```python
from build123d import *

# Parameters (mm, degrees)
SKETCH1_R           = 3.5
BOSS_EXTRUDE1_DEPTH = 30
SKETCH2_R           = 1.2
CUT_EXTRUDE1_DEPTH  = 15
SKETCH3_R           = 1.1
CUT_EXTRUDE2_DEPTH  = 15
CUT_EXTRUDE3_START  = -30
CUT_EXTRUDE3_DEPTH  = 30


with BuildPart() as part:
    # Sketch1 → Boss-Extrude1 (new body)
    with BuildSketch(Plane(origin=(0, 0, 0), x_dir=(0, 0, -1), z_dir=(1, 0, 0))):
        Circle(SKETCH1_R)
    extrude(amount=BOSS_EXTRUDE1_DEPTH)

    # Sketch2 → Cut-Extrude1 (cut)
    with BuildSketch(Plane.ZY):
        Circle(SKETCH2_R)
    extrude(amount=-CUT_EXTRUDE1_DEPTH, mode=Mode.SUBTRACT)

    # Sketch3 → Cut-Extrude2 (cut)
    with BuildSketch(Plane(origin=(30, 0, 0), x_dir=(0, 0, -1), z_dir=(1, 0, 0))):
        Circle(SKETCH3_R)
    extrude(amount=-CUT_EXTRUDE2_DEPTH, mode=Mode.SUBTRACT)

    # Sketch4 → Cut-Extrude3 (cut)
    with BuildSketch(Plane(origin=(30, 0, 0), x_dir=(0, 0, -1), z_dir=(1, 0, 0)).offset(CUT_EXTRUDE3_START)):
        with BuildLine():
            Line((2.449489743, 2.5), (2.449489743, -2.5))
            ThreePointArc((2.449489743, -2.5), (3.5, 0), (2.449489743, 2.5))
        make_face()
    extrude(amount=CUT_EXTRUDE3_DEPTH, mode=Mode.SUBTRACT)


solid = part.part
```
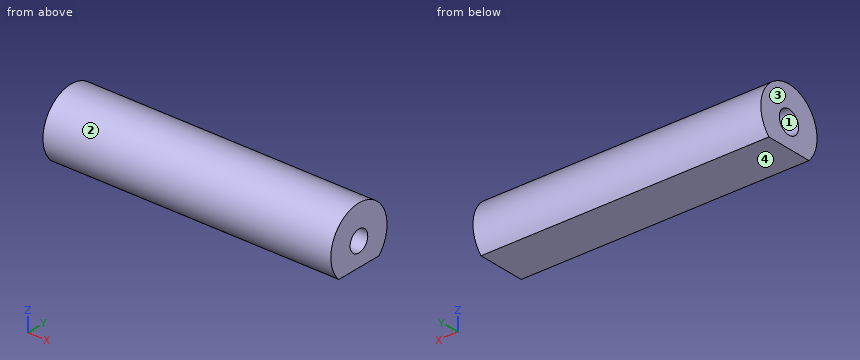
Input: part model. Units: mm. Frame: model coordinates. Face numbers are marked on the shaded views. Round coordinates to 2 decimals unless told otherwise and drop trailing zeros. Loops run counter-clockwise (first coordinate to the right, second up) from the corner with the lowest first, then second, coordinate; pieces in that order, holes last. Notation, with made-up numbers: (78.5, -37.75) -> (113.5, -37.75) arc R17 cw to (113.5, -16.75) -> close; hole circle Ø3 at (-25, 43). An arc over 180 degrees is marked (long way). Use one line per item in the form item = value. Start each with the question number.
Item 1: Section query A-A on z = 0. Return the cut outline in (x, y), then the cut area to 3 significant figures.
Item 2: Contact query for a flat-ended pin moving along its axis: pin 1 Ø2 at (x, z) = (9.5, 1.5) entering from -Y. Output: stop coordinate, or through.
Item 3: Section query C-C on x = 23.5. Return the cut outline in (y, z), then the cut area to 3 significant figures.
Item 4: Material intervals for L1, parallel to Y at x = 25.5, z = 0; L2, parallel to Y at x = 6.25, z = 0; L3, parallel to Z at x = 18, y = -0.25, sorted ascending. Write a range as from..to.
Item 5: Mould query, pull axis Z, two halves, no side actions, for the marked faces 1, 2, 3 and 4. Classes: pulls with the +Z half, pulls with the -Z half, needs draft (parallel to the pull), parting line crosses it, or undercut.
Item 6: Section query D-D on z = -1.8. Return the cut outline in (x, y), then the cut area to 3 significant figures.
Item 7: Section query B-B on x = 10.75. Return the cut outline in (y, z), then the cut area to 3 significant figures.
Ans:
q1.outline = (0, -3.5) -> (30, -3.5) -> (30, -1.1) -> (15, -1.1) -> (15, -1.2) -> (0, -1.2) -> close; (0, 1.2) -> (15, 1.2) -> (15, 1.1) -> (30, 1.1) -> (30, 3.5) -> (0, 3.5) -> close
q1.area = 141 mm^2
q2.pin_1 = -3.46
q3.outline = (-2.5, -2.45) -> (2.5, -2.45) arc R3.5 ccw (long way) to start; hole circle Ø2.2 at (0, 0)
q3.area = 31.1 mm^2
q4.L1 = -3.5..-1.1, 1.1..3.5
q4.L2 = -3.5..-1.2, 1.2..3.5
q4.L3 = -2.45..-1.07, 1.07..3.49
q5.face_1 = undercut
q5.face_2 = parting line crosses it
q5.face_3 = needs draft
q5.face_4 = pulls with the -Z half
q6.outline = (0, -3) -> (30, -3) -> (30, 3) -> (0, 3) -> close
q6.area = 180 mm^2
q7.outline = (-2.5, -2.45) -> (2.5, -2.45) arc R3.5 ccw (long way) to start; hole circle Ø2.4 at (0, 0)
q7.area = 30.3 mm^2
